Check sheet for the drawn part. Datum: minimum x, y, z corner. Units: mm. A direction names the side the tool comes from. Coordinates: 2 decimals unless noted, no trailing zeros. Order: outer loops, then holes, each group sorted by start corner. A loop starts at its lowest first (then second) coordinate and runs counter-clockwise, first axis right, second up. Notation, with made-up numbers: (34.25, -14.75) -> (83.25, -14.75) arc R22 cw to (83.25, -2.75) -> close; hole circle Ø8 at (-34, -27.75). An arc over 180 degrees is marked (long way). Answer as CSV lines item,"result".
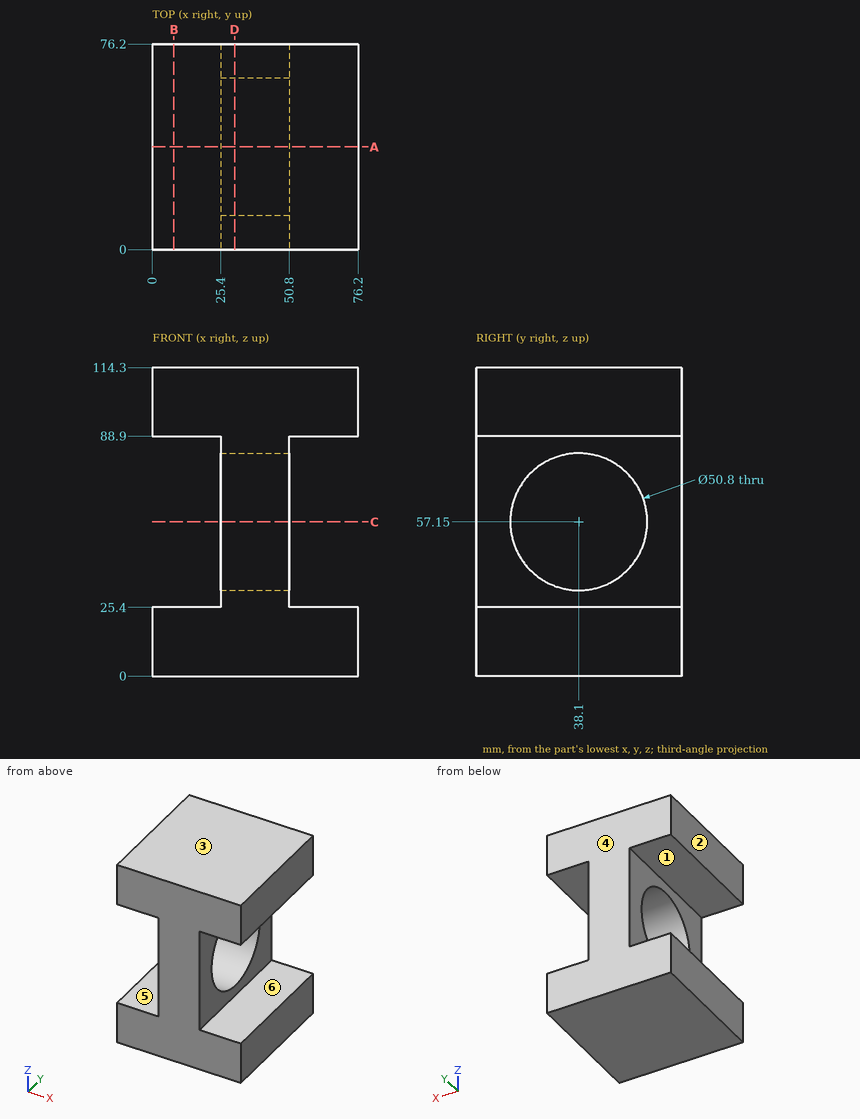
Item 1: Release check for a two-part mould opening along Z. For the marked faces 1, 2 and 3 record: +Z half, -Z half, draft (parallel to the pull), parting line (faces both ways), or undercut.
Answer list:
face 1,"undercut"
face 2,"draft"
face 3,"+Z half"
Item 2: Section check D-D, the plane x = 30.5. Record the boundary of the cut face in (y, z).
Answer list:
outline,"(0, 0) -> (76.2, 0) -> (76.2, 114.3) -> (0, 114.3) -> close; hole circle Ø50.8 at (38.1, 57.15)"
Item 3: Section check A-A, the plane y = 38.1. Record the boundary of the cut face in (x, z).
Answer list:
outline,"(0, 0) -> (76.2, 0) -> (76.2, 25.4) -> (50.8, 25.4) -> (50.8, 31.75) -> (25.4, 31.75) -> (25.4, 25.4) -> (0, 25.4) -> close; (0, 88.9) -> (25.4, 88.9) -> (25.4, 82.55) -> (50.8, 82.55) -> (50.8, 88.9) -> (76.2, 88.9) -> (76.2, 114.3) -> (0, 114.3) -> close"
Item 4: Tool access check on the marked faces 4, 5 and 6. Record the directions out of +Z, -Z, +X, -X, +Y, -Y that give a thin tool (end or side, any length) a straight path to the whole face; none if there is none.
Answer list:
face 4,"+Z, -Z, +X, -X, +Y"
face 5,"-X, +Y, -Y"
face 6,"+X, +Y, -Y"
Item 5: Thickness scan on line 1 (Y direction, x = 32, z = 57); line 2 (Z direction, x = 64.5, y = 37.5); line 3 (Z direction, x = 41, y = 38). Record the ranges inside material, lowest first.
Answer list:
line 1,"0 to 12.7, 63.5 to 76.2"
line 2,"0 to 25.4, 88.9 to 114.3"
line 3,"0 to 31.75, 82.55 to 114.3"
Item 6: Section check B-B, the plane x = 8. Record the boundary of the cut face in (y, z), plus the area to 3 significant figures.
Answer list:
outline,"(0, 0) -> (76.2, 0) -> (76.2, 25.4) -> (0, 25.4) -> close; (0, 88.9) -> (76.2, 88.9) -> (76.2, 114.3) -> (0, 114.3) -> close"
area,"3,870 mm2"
Item 7: Section check C-C, the plane z = 57.15. Record the boundary of the cut face in (x, y).
Answer list:
outline,"(25.4, 0) -> (50.8, 0) -> (50.8, 12.7) -> (25.4, 12.7) -> close; (25.4, 63.5) -> (50.8, 63.5) -> (50.8, 76.2) -> (25.4, 76.2) -> close"
Item 8: Depth check by flat-ended pin: pin 1 Ø5 at (y, z) = (9, 44.5) entering from -X; pin 2 Ø10 at (y, z) = (23, 27) entering from -X; pin 3 Ø4 at (y, z) = (14.5, 51) entering from +X. Enter the tip coordinate at first touch or a pass-through.
Answer list:
pin 1,"x = 25.4"
pin 2,"x = 0"
pin 3,"x = 50.8"
